Could you check a few things on this drawing? It's one solid part, dimensions in mm from its lowest x, y, z. Round coordinates to 2 decimals unless told otherwise and drop trailing zeros. Write each loop counter-clockwise with the first axis right and the second up, starting at its lowest first coordinate (ties: lowest second). Pieces come first, ordered by that corner, then holes. Notation, with made-up numbers: (41.5, -32) -> (76.5, -32) arc R11 ccw to (76.5, -24) -> close; hole circle Ø3 at (41, 50). An arc over 180 degrees is marked (long way). Return JSON: item names as keys, results as strings.
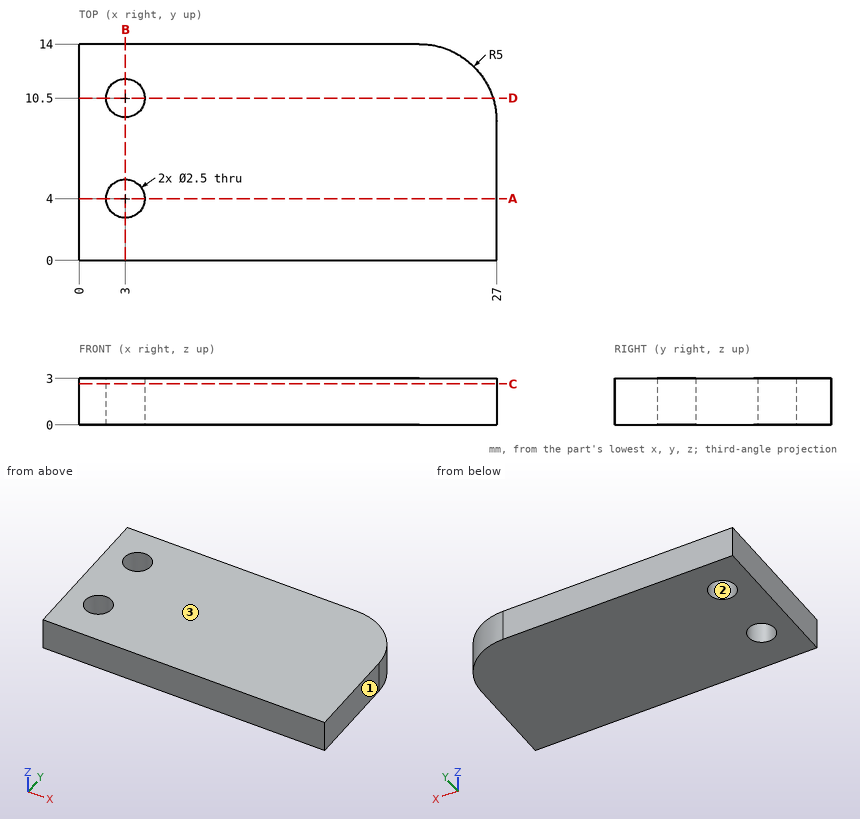
1) I want a section at D-D, the plane y = 10.5. Please give me the cut outline in (x, z), and give its area (3 significant figures).
Return value:
{"outline": "(0, 0) -> (1.75, 0) -> (1.75, 3) -> (0, 3) -> close; (4.25, 0) -> (26.77, 0) -> (26.77, 3) -> (4.25, 3) -> close", "area": "72.8 mm²"}
2) Thinking about a two-plate mould opening in X: for the marked faces 1, 2 and 3, which applies, pulls with the +X half, pulls with the -X half, needs draft (parallel to the pull), parting line crosses it, or undercut?
Return value:
{"face 1": "pulls with the +X half", "face 2": "undercut", "face 3": "needs draft"}
3) I want a section at A-A, the plane y = 4. Please give me the cut outline in (x, z), and give its area (3 significant figures).
Return value:
{"outline": "(0, 0) -> (1.75, 0) -> (1.75, 3) -> (0, 3) -> close; (4.25, 0) -> (27, 0) -> (27, 3) -> (4.25, 3) -> close", "area": "73.5 mm²"}
4) If I drill on probe 1 along Y at (x, z) = (3, 1.9); probe 2 along X at (y, z) = (11, 1.3); probe 3 along X at (y, z) = (4.75, 2.2), over which ranges is the centre line in solid material (lowest first)? Write a range as [from, to].
Return value:
{"probe 1": "[0, 2.75], [5.25, 9.25], [11.75, 14]", "probe 2": "[0, 1.85], [4.15, 26.58]", "probe 3": "[0, 2], [4, 27]"}
5) Will this pin go through, and if not, where does the flat tip stop? pin 1 Ø2 at (x, y) = (3, 4) entering from +Z.
Return value:
{"pin 1": "through"}
6) I want a section at B-B, the plane x = 3. Please give me the cut outline in (y, z), and give its area (3 significant figures).
Return value:
{"outline": "(0, 0) -> (2.75, 0) -> (2.75, 3) -> (0, 3) -> close; (5.25, 0) -> (9.25, 0) -> (9.25, 3) -> (5.25, 3) -> close; (11.75, 0) -> (14, 0) -> (14, 3) -> (11.75, 3) -> close", "area": "27.0 mm²"}
7) I want a section at C-C, the plane z = 2.65. Please give me the cut outline in (x, y), and give its area (3 significant figures).
Return value:
{"outline": "(0, 0) -> (27, 0) -> (27, 9) arc R5 ccw to (22, 14) -> (0, 14) -> close; hole circle Ø2.5 at (3, 4); hole circle Ø2.5 at (3, 10.5)", "area": "363 mm²"}
